Verification items for the finished model (mm, model axes). A direction names the side the tool comes from. Round coordinates to 2 decimals unless told otherwise and drop trailing zeros. Write each loop counter-clockwise with the first axis right and the second up, starting at its lowest first coordinate (ties: lowest second). Pieces come first, ordered by that corner, then holes. Notation, with made-up numbers: (-38, 41.25) -> (1, 41.25) arc R23 ccw to (1, 73.25) -> close; hole circle Ø5 at (-17, -16.5). An arc over 180 degrees is marked (long way). Use CSV: the item, a comma, the result in double quotes.
```python
from build123d import *

# Parameters (mm, degrees)
F0_W        = 40
F0_H        = 40
F1_DEPTH    = 2
F2_T1_DEPTH = 65.7293606605
F2_T3_DEPTH = 65.7293606605
F3_D        = 3.3
F4_W        = 4.3
F4_H        = 9
F5_DEPTH    = 25
F6_W        = 32
F6_H        = 32
F7_DEPTH    = 1.5


# Not quite as in the source:
# - a fillet or chamfer that OpenCascade refuses, or shapes differently, is made with other operations: its cross-section is extruded or revolved along the edge and cut away or added


with BuildPart() as f1:
    # F0 (on Top) → F1 (new body)
    with BuildSketch(Plane.XY):
        with Locations((0.9159009159, 13.0545736344)):
            Rectangle(F0_W, F0_H)
    extrude(amount=F1_DEPTH)

    # F2: fillet of radius 7.62 on 4 edges, made by hand

    # F2_s2 → F2_t1 (cut)
    with BuildSketch(Plane.XZ.offset(-45.9192539647)):
        with BuildLine():
            ThreePointArc((-19.0840990841, 0), (-16.6986617004, 1.4824221221), (-13.938226952, 2))
            Line((-13.938226952, 2), (-19.0840990841, 2))
            Line((-19.0840990841, 2), (-19.0840990841, 0))
        make_face()
        with BuildLine():
            ThreePointArc((20.9159009159, 0), (18.5304635321, 1.4824221221), (15.7700287838, 2))
            Line((15.7700287838, 2), (20.9159009159, 2))
            Line((20.9159009159, 2), (20.9159009159, 0))
        make_face()
    extrude(amount=F2_T1_DEPTH, mode=Mode.SUBTRACT)

    # F2_s4 → F2_t3 (cut)
    with BuildSketch(Plane.YZ.offset(-31.9487794144)):
        with BuildLine():
            ThreePointArc((-6.9454263656, 0), (-4.5599889818, 1.4824221221), (-1.7995542335, 2))
            Line((-1.7995542335, 2), (-6.9454263656, 2))
            Line((-6.9454263656, 2), (-6.9454263656, 0))
        make_face()
        with BuildLine():
            ThreePointArc((33.0545736344, 0), (30.6691362507, 1.4824221221), (27.9087015023, 2))
            Line((27.9087015023, 2), (33.0545736344, 2))
            Line((33.0545736344, 2), (33.0545736344, 0))
        make_face()
    extrude(amount=F2_T3_DEPTH, mode=Mode.SUBTRACT)

    # F3 (through all)
    with Locations(Plane(origin=(0, 0, 0), x_dir=(1, 0, 0), z_dir=(0, 0, -1))):
        with Locations((-16.5840990841, 4.4454263656), (-16.5840990841, -30.5545736344), (18.4159009159, -30.5545736344), (18.4159009159, 4.4454263656)):
            Hole(F3_D / 2)

    # F4 (on Top) → F5 (cut)
    with BuildSketch(Plane.XY):
        with Locations((-11.0940990841, 14.1945736344)):
            Rectangle(F4_W, F4_H)
    extrude(amount=F5_DEPTH, mode=Mode.SUBTRACT)

    # F6 (on Top) → F7 (cut)
    with BuildSketch(Plane.XY):
        with Locations((0.9159009159, 13.0545736344)):
            Rectangle(F6_W, F6_H)
    extrude(amount=F7_DEPTH, mode=Mode.SUBTRACT)


solid = f1.part
```
Q1. Go/stop test with flat-tipped pins: P1, Ø9.5, axis at x = 1.5, y = 15.5, coming from the -Z side; P2, Ø5.5, axis at x = 18.42, y = -4.45, coming from the +Z side; P3, Ø4, axis at x = -16.58, y = -4.45, coming from the +Z side; P4, Ø3, axis at x = -16.58, y = 30.55, coming from the +Z side. Record where each tip stops, or that it passes through.
Filled in:
P1,"z = 1.5"
P2,"z = 1.97"
P3,"z = 1.9"
P4,"through"
Q2. Section check A-A (y = 12). Record the cut outline in (x, z).
Filled in:
outline,"(-19.08, 0) -> (-15.08, 0) -> (-15.08, 1.5) -> (-13.24, 1.5) -> (-13.24, 2) -> (-13.94, 2) arc R7.62 ccw to start; (-8.94, 1.5) -> (16.92, 1.5) -> (16.92, 0) -> (20.92, 0) arc R7.62 ccw to (15.77, 2) -> (-8.94, 2) -> close"
Q3. Material ranges on L1, parallel to X at y = -5, z = 0.2; L2, parallel to Y at x = -16, z = 0.6; L3, parallel to Y at x = -2.5, z = 0.25, recorded low to high.
Filled in:
L1,"-18.86 to -18.14, -15.03 to 16.86, 19.97 to 20.69"
L2,"-6.2 to -5.99, -2.9 to 29.01, 32.1 to 32.31"
L3,"-6.66 to -2.95, 29.05 to 32.77"
Q4. Access from +Z, -Z, +X, -X, +Y, -Y to the whole of each face (thin tool, end or side, straight path). Record for faces 1 (the flat face through (1, -2.945, 1)), 2 (the cylindrical face through (17.529, 29.163, 0.734)).
Filled in:
face 1,"-Z"
face 2,"+Z, -Z"
Q5. Mould release check, pull along Y, two halves, no side actions. Record for faces 3 (the cylindrical face through (0.636, -4.597, 1.468)), 4 (the cylindrical face through (0.636, 30.706, 1.468)), 5 (the cylindrical face through (-15.275, -3.441, 0.734)): released by +Y, released by -Y, zero draft, split by the parting line, or undercut.
Filled in:
face 3,"released by -Y"
face 4,"released by +Y"
face 5,"undercut"
Q6. Section check B-B (x = 11.5). Record the cut outline in (y, z).
Filled in:
outline,"(-6.95, 0) -> (-2.95, 0) -> (-2.95, 1.5) -> (29.05, 1.5) -> (29.05, 0) -> (33.05, 0) arc R7.62 ccw to (27.91, 2) -> (-1.8, 2) arc R7.62 ccw to start"
Q7. Section check C-C (y = 25.5). Record the cut outline in (x, z).
Filled in:
outline,"(-19.08, 0) -> (-15.08, 0) -> (-15.08, 1.5) -> (16.92, 1.5) -> (16.92, 0) -> (20.92, 0) arc R7.62 ccw to (15.77, 2) -> (-13.94, 2) arc R7.62 ccw to start"
